```python
from build123d import *

# Parameters (mm, degrees)
REVOLVE1_ANGLE     = 270
CUT_EXTRUDE3_START = -120
CUT_EXTRUDE3_DEPTH = 120


# Read off the part's stored shape, not the designer's step: Cut-Extrude3
with BuildPart() as part:
    # Sketch1 → Revolve1 (revolve)
    with BuildSketch(Plane.XY):
        Polygon((-141.986286211, 15), (-21.986286211, 15), (-21.986286211, 30), (-93.986286211, 30), (-93.986286211, 47), (-53.986286211, 47), (-53.986286211, 62), (-13.986286211, 62), (-13.986286211, 77), (18.013713789, 77), (18.013713789, 85), (-21.986286211, 85), (-21.986286211, 70), (-61.986286211, 70), (-61.986286211, 55), (-101.986286211, 55), (-101.986286211, 40), (-141.986286211, 40), align=None)
    revolve(axis=Axis((-141.986286211, 0, 0), (1, 0, 0)), revolution_arc=REVOLVE1_ANGLE)

    # Cut-Extrude3 outline → Cut-Extrude3 (cut)
    with BuildSketch(Plane.ZY.offset(141.986286211).offset(CUT_EXTRUDE3_START)):
        with BuildLine():
            Line((14.774482913, -2.591265069), (21, -2.591265069))
            Line((21, -2.591265069), (21, 3.408734931))
            Line((21, 3.408734931), (14.607550314, 3.408734931))
            ThreePointArc((14.607550314, 3.408734931), (14.994197849, 0.41717007), (14.774482913, -2.591265069))
        make_face()
    extrude(amount=CUT_EXTRUDE3_DEPTH, mode=Mode.SUBTRACT)


solid = part.part
```
For this review, take the finished solid that the model builds, in its own axes (mm). A direction names the side the tool comes from. Coordinates: 2 decimals unless noted, no trailing zeros. Loops run counter-clockwise (first coordinate to the right, second up) from the corner with the lowest first, then second, coordinate; pieces in that order, holes last. Notation, with made-up numbers: (-30, 75.25) -> (-1, 75.25) arc R22 cw to (-1, 97.25) -> close; hole circle Ø8 at (55.25, 9.25). An arc over 180 degrees is marked (long way). Return JSON: item names as keys, results as strings. Group by question number.
(1) Consider section A-A, the plane x = -73. Give the boundary of the cut face in (y, z).
(2) For pin 1 Ø1.5 at (x, y) = (-71, 8.5) entering from -Z; pin 2 Ø1.5 at (x, y) = (-64, 54) entering from -Z; pin 3 Ø12 at (y, z) = (-38.5, -27.5) entering from -X, all flat-tipped, find the tip position at first contact; note any pin that passes through.
(3) Mouldability with a two-part tool opening along Z and no side actions: class faces 1 (the cylindrical face through (-122.27, -27.34, 29.2)), 2 (the cylindrical face through (-33.706, -42.371, 45.263)), 3 (the flat face through (-141.986, -18, 1)), 4 (the cylindrical face through (2.238, -52.622, 56.213)) as pulls with the +Z half, pulls with the -Z half, needs draft (parallel to the pull), parting line crosses it, or undercut.
(4) To check wall thickness, follow L1, parallel to X at y = -22.5, z = -55.5; L2, parallel to Y at x = -5.5, z = 62; L3, parallel to Z at x = -74, y = 9.5. State the ranges of each line that lie inside material, in increasing order.
(5) Consider section B-B, the plane y = -67. Give the boundary of the cut face in (x, z), plus the area to 3 significant figures.
(6) Tool access review of faces 5 (the flat face through (-81, 3.409, 18)), 6 (the cylindrical face through (-73.71, -32.12, 34.31)), 7 (the flat face through (-81, -2.591, 18)), 8 (the flat face through (-61.986, -42, 37)), 9 (the flat face through (18.014, -56, 57)): name each direction out of +Z, -Z, +X, -X, +Y, -Y from which nothing blocks a thin tool from reaching the whole face with its end or side.
(7) Consider section D-D, the plane x = -6. Give the boundary of the cut face in (y, z), plus the area to 3 significant figures.
(8) Consider section C-C, the plane z = -43.5. Give the boundary of the cut face in (x, y), plus the area to 3 significant figures.
Results below:
{
 "1": {"outline": "(-2.59, 14.77) -> (-2.59, 21) -> (3.41, 21) -> (3.41, 14.61) arc R15 cw to (15, 0) -> (30, 0) arc R30 ccw (long way) to (0, -30) -> (0, -15) arc R15 cw to start; (0, -55) -> (0, -47) arc R47 cw (long way) to (47, 0) -> (55, 0) arc R55 ccw (long way) to start"},
 "2": {"pin 1": "stops at z = 11.81", "pin 2": "stops at z = 0", "pin 3": "stops at x = -101.99"},
 "3": {"face 1": "parting line crosses it", "face 2": "undercut", "face 3": "needs draft", "face 4": "undercut"},
 "4": {"L1": "x = -61.99 to -53.99", "L2": "y = -58.15 to -45.66, 45.66 to 58.15", "L3": "z = 11.61 to 28.46, 46.03 to 54.17"},
 "5": {"outline": "(-61.99, -20.27) -> (-21.99, -20.27) -> (-21.99, -52.31) -> (18.01, -52.31) -> (18.01, -37.95) -> (-13.99, -37.95) -> (-13.99, 37.95) -> (18.01, 37.95) -> (18.01, 52.31) -> (-21.99, 52.31) -> (-21.99, 20.27) -> (-61.99, 20.27) -> close", "area": "3,380 mm2"},
 "6": {"face 5": "-Z, +X, -X", "face 6": "+X", "face 7": "+X, -X", "face 8": "-X", "face 9": "+Z, -Z, +X, +Y, -Y"},
 "7": {"outline": "(0, -85) -> (0, -77) arc R77 cw (long way) to (77, 0) -> (85, 0) arc R85 ccw (long way) to start", "area": "3,050 mm2"},
 "8": {"outline": "(-101.99, -33.66) -> (-61.99, -33.66) -> (-61.99, -54.84) -> (-21.99, -54.84) -> (-21.99, -73.03) -> (18.01, -73.03) -> (18.01, -63.54) -> (-13.99, -63.54) -> (-13.99, -44.18) -> (-53.99, -44.18) -> (-53.99, -17.8) -> (-93.99, -17.8) -> (-93.99, 0) -> (-101.99, 0) -> close", "area": "1,950 mm2"}
}
